```python
from build123d import *

# Parameters (mm, degrees)
SKETCH_2_W                 = 432
SKETCH_2_H                 = 330
EXTRUDE_1_DEPTH            = 4
FILLET_1_R                 = 2
HOLE_WIZARD_M4_AT_2_COUNT  = 2
HOLE_WIZARD_M4_AT_2_PITCH  = 124
HOLE_WIZARD_M4_AT_3_COUNT  = 2
HOLE_WIZARD_M4_AT_3_PITCH  = 248
HOLE_WIZARD_M4_AT_4_COUNT  = 2
HOLE_WIZARD_M4_AT_4_PITCH  = 372
HOLE_WIZARD_M4_AT_5_COUNT  = 2
HOLE_WIZARD_M4_AT_5_PITCH  = 397.256214552
HOLE_WIZARD_M4_AT_6_COUNT  = 2
HOLE_WIZARD_M4_AT_6_PITCH  = 412.701465953
HOLE_WIZARD_M4_AT_7_COUNT  = 2
HOLE_WIZARD_M4_AT_7_PITCH  = 446.130586264
HOLE_WIZARD_M4_AT_8_COUNT  = 2
HOLE_WIZARD_M4_AT_8_PITCH  = 493.905355306
HOLE_WIZARD_M4_AT_9_COUNT  = 2
HOLE_WIZARD_M4_AT_9_PITCH  = 489.070802645
HOLE_WIZARD_M4_AT_10_COUNT = 2
HOLE_WIZARD_M4_AT_10_PITCH = 402.87746276
HOLE_WIZARD_M4_AT_11_COUNT = 2
HOLE_WIZARD_M4_AT_11_PITCH = 340.855174524
HOLE_WIZARD_M4_AT_12_COUNT = 2
HOLE_WIZARD_M4_AT_12_PITCH = 317.5
HOLE_WIZARD_M4_AT_13_COUNT = 2
HOLE_WIZARD_M4_AT_13_PITCH = 295.517342977
HOLE_WIZARD_M4_AT_14_COUNT = 2
HOLE_WIZARD_M4_AT_14_PITCH = 205.962375205
HOLE_WIZARD_M4_AT_15_COUNT = 2
HOLE_WIZARD_M4_AT_15_PITCH = 117.091844293
HOLE_WIZARD_M4_AT_16_COUNT = 2
HOLE_WIZARD_M4_AT_16_PITCH = 34.648232278


with BuildPart() as part:
    # 草圖2 → 填料-伸長1 (new body)
    with BuildSketch(Plane(origin=(0, 0, 0), x_dir=(1, 0, 0), z_dir=(0, 1, 0))):
        with Locations((216, 165)):
            Rectangle(SKETCH_2_W, SKETCH_2_H)
    extrude(amount=EXTRUDE_1_DEPTH)

    # 圓角1
    fillet_1_edges = [part.edges().sort_by_distance(p)[0] for p in [
        (216, 4, 0),
    ]]
    fillet(fillet_1_edges, radius=FILLET_1_R)

    # 草圖4 → M4 測板連接 (revolve, cut)
    with BuildSketch(Plane(origin=(30, 4, -324.5), x_dir=(0, 0, 1), z_dir=(1, 0, 0))):
        Polygon((0, 0), (0, 4), (2.25, 4), (2.25, 2.45), (4.7, 0), align=None)
    hole_wizard_m4 = revolve(axis=Axis((30, 10.35, -324.5), (0, -1, 0)), mode=Mode.SUBTRACT)

    # M4 測板連接 at 2: M4 測板連接 ×2
    with Locations(*[(i * HOLE_WIZARD_M4_AT_2_PITCH, 0, 0) for i in range(1, HOLE_WIZARD_M4_AT_2_COUNT)]):
        add(hole_wizard_m4, mode=Mode.SUBTRACT)

    # M4 測板連接 at 3: M4 測板連接 ×2
    with Locations(*[(i * HOLE_WIZARD_M4_AT_3_PITCH, 0, 0) for i in range(1, HOLE_WIZARD_M4_AT_3_COUNT)]):
        add(hole_wizard_m4, mode=Mode.SUBTRACT)

    # M4 測板連接 at 4: M4 測板連接 ×2
    with Locations(*[(i * HOLE_WIZARD_M4_AT_4_PITCH, 0, 0) for i in range(1, HOLE_WIZARD_M4_AT_4_COUNT)]):
        add(hole_wizard_m4, mode=Mode.SUBTRACT)

    # M4 測板連接 at 5: M4 測板連接 ×2
    with Locations(*[Vector(0.998096406, 0, 0.061673044) * (i * HOLE_WIZARD_M4_AT_5_PITCH) for i in range(1, HOLE_WIZARD_M4_AT_5_COUNT)]):
        add(hole_wizard_m4, mode=Mode.SUBTRACT)

    # M4 測板連接 at 6: M4 測板連接 ×2
    with Locations(*[Vector(0.960742892, 0, 0.277440255) * (i * HOLE_WIZARD_M4_AT_6_PITCH) for i in range(1, HOLE_WIZARD_M4_AT_6_COUNT)]):
        add(hole_wizard_m4, mode=Mode.SUBTRACT)

    # M4 測板連接 at 7: M4 測板連接 ×2
    with Locations(*[Vector(0.888753231, 0, 0.458385967) * (i * HOLE_WIZARD_M4_AT_7_PITCH) for i in range(1, HOLE_WIZARD_M4_AT_7_COUNT)]):
        add(hole_wizard_m4, mode=Mode.SUBTRACT)

    # M4 測板連接 at 8: M4 測板連接 ×2
    with Locations(*[Vector(0.802785383, 0, 0.596268084) * (i * HOLE_WIZARD_M4_AT_8_PITCH) for i in range(1, HOLE_WIZARD_M4_AT_8_COUNT)]):
        add(hole_wizard_m4, mode=Mode.SUBTRACT)

    # M4 測板連接 at 9: M4 測板連接 ×2
    with Locations(*[Vector(0.760626065, 0, 0.649190257) * (i * HOLE_WIZARD_M4_AT_9_PITCH) for i in range(1, HOLE_WIZARD_M4_AT_9_COUNT)]):
        add(hole_wizard_m4, mode=Mode.SUBTRACT)

    # M4 測板連接 at 10: M4 測板連接 ×2
    with Locations(*[Vector(0.615571788, 0, 0.788080817) * (i * HOLE_WIZARD_M4_AT_10_PITCH) for i in range(1, HOLE_WIZARD_M4_AT_10_COUNT)]):
        add(hole_wizard_m4, mode=Mode.SUBTRACT)

    # M4 測板連接 at 11: M4 測板連接 ×2
    with Locations(*[Vector(0.363790869, 0, 0.931480651) * (i * HOLE_WIZARD_M4_AT_11_PITCH) for i in range(1, HOLE_WIZARD_M4_AT_11_COUNT)]):
        add(hole_wizard_m4, mode=Mode.SUBTRACT)

    # M4 測板連接 at 12: M4 測板連接 ×2
    with Locations(*[(0, 0, i * HOLE_WIZARD_M4_AT_12_PITCH) for i in range(1, HOLE_WIZARD_M4_AT_12_COUNT)]):
        add(hole_wizard_m4, mode=Mode.SUBTRACT)

    # M4 測板連接 at 13: M4 測板連接 ×2
    with Locations(*[Vector(-0.082905456, 0, 0.996557417) * (i * HOLE_WIZARD_M4_AT_13_PITCH) for i in range(1, HOLE_WIZARD_M4_AT_13_COUNT)]):
        add(hole_wizard_m4, mode=Mode.SUBTRACT)

    # M4 測板連接 at 14: M4 測板連接 ×2
    with Locations(*[Vector(-0.118953765, 0, 0.992899794) * (i * HOLE_WIZARD_M4_AT_14_PITCH) for i in range(1, HOLE_WIZARD_M4_AT_14_COUNT)]):
        add(hole_wizard_m4, mode=Mode.SUBTRACT)

    # M4 測板連接 at 15: M4 測板連接 ×2
    with Locations(*[Vector(-0.209237459, 0, 0.977864861) * (i * HOLE_WIZARD_M4_AT_15_PITCH) for i in range(1, HOLE_WIZARD_M4_AT_15_COUNT)]):
        add(hole_wizard_m4, mode=Mode.SUBTRACT)

    # M4 測板連接 at 16: M4 測板連接 ×2
    with Locations(*[Vector(-0.707106781, 0, 0.707106781) * (i * HOLE_WIZARD_M4_AT_16_PITCH) for i in range(1, HOLE_WIZARD_M4_AT_16_COUNT)]):
        add(hole_wizard_m4, mode=Mode.SUBTRACT)


solid = part.part
```
Could you check a few things on this model? Use its own coordinates, in mm. Coordinates: 2 decimals unless noted, no trailing zeros. Use a Markdown table: item, result.
Q1. Thinking about a two-plate mould opening in Z: for faces 1 (the flat face through (213, 4, -168)), 2 (the conical face through (153.9, 1.7, -326.9)), 3 (the conical face through (5.4, 1.7, -302.4)), which applies, +Z half, -Z half, draft (parallel to the pull), parting line (faces both ways), or undercut?
Geometry check:
| item | result |
|---|---|
| face 1 | draft |
| face 2 | undercut |
| face 3 | undercut |
Q2. Please list where these lines run through material, in increasing order: L1, parallel to X at y = 0.55, z = -324.5; L2, parallel to X at y = 1, z = -210; L3, parallel to Z at x = 404, y = 2.3.
Geometry check:
| item | result |
|---|---|
| L1 | x = 0 to 27.75, 32.25 to 151.75, 156.25 to 275.75, 280.25 to 399.75, 404.25 to 432 |
| L2 | x = 0 to 3.25, 7.75 to 424.25, 428.75 to 432 |
| L3 | z = -330 to -326.74, -322.26 to -9.24, -4.76 to -0.02 |
Q3. I'm going to push flat-ended pins straight in: pin 1 Ø5 at (x, z) = (402, -7) entering from +Y; pin 2 Ø6 at (x, z) = (402, -324.5) entering from +Y. Where does each tip first touch, or does it pass through?
Geometry check:
| item | result |
|---|---|
| pin 1 | stops at y = 1.8 |
| pin 2 | stops at y = 2.3 |
